Read the model definition and answer for the solid it produces. Units are mm, in the model's axes. A direction names the side the tool comes from. Give positions to 0.01 mm unless a question says otherwise; leave off trailing zeros. Order: outer loops, then holes, each group sorted by start corner. A loop starts at its lowest first (then second) coordinate and runs counter-clockwise, first axis right, second up. Notation, with made-up numbers: M 64,22.25 L 71,22.25 A32 ccw 71,51.25 Z; hole C -23.75,-14 d11. An arc over 180 degrees is marked long. One line per item, written item: value.
from build123d import *

# Parameters (mm, degrees)
SKETCH1_W                = 4
SKETCH1_H                = 15
BOSS_EXTRUDE1_DEPTH      = 4
SKETCH2_R                = 0.925
BOSS_EXTRUDE2_DEPTH      = 2
BOSS_EXTRUDE2_DEPTH_BACK = 17
CHAMFER1_SIZE            = 0.5
BOSS_EXTRUDE3_DEPTH      = 2
BOSS_EXTRUDE4_DEPTH      = 2


with BuildPart() as part:
    # Sketch1 → Boss-Extrude1 (new body)
    with BuildSketch(Plane(origin=(0, 0, 0), x_dir=(1, 0, 0), z_dir=(0, 1, 0))):
        Rectangle(SKETCH1_W, SKETCH1_H)
    extrude(amount=BOSS_EXTRUDE1_DEPTH)

    # Sketch2 → Boss-Extrude2 (add, two sides)
    with BuildSketch(Plane.XY.offset(7.5)) as boss_extrude2_sk:
        with Locations((0, 2)):
            Circle(SKETCH2_R)
    extrude(amount=BOSS_EXTRUDE2_DEPTH)
    extrude(boss_extrude2_sk.sketch, amount=-BOSS_EXTRUDE2_DEPTH_BACK)

    # Chamfer1
    chamfer1_edges = [part.edges().sort_by_distance(p)[0] for p in [
        (-2, 4, 0),
        (2, 4, 0),
        (-2, 0, 0),
        (2, 0, 0),
    ]]
    chamfer(chamfer1_edges, length=CHAMFER1_SIZE)

    # Sketch3 → Boss-Extrude3 (add)
    with BuildSketch(Plane.XY.offset(9.5)):
        with BuildLine():
            Line((-0.75, 2.925), (0.75, 2.925))
            ThreePointArc((0.75, 2.925), (1.675, 2), (0.75, 1.075))
            Line((0.75, 1.075), (-0.75, 1.075))
            ThreePointArc((-0.75, 1.075), (-1.675, 2), (-0.75, 2.925))
        make_face()
    extrude(amount=BOSS_EXTRUDE3_DEPTH)

    # Sketch4 → Boss-Extrude4 (add)
    with BuildSketch(Plane(origin=(0, 0, -9.5), x_dir=(-1, 0, 0), z_dir=(0, 0, -1))):
        with BuildLine():
            Line((-0.75, 2.925), (0.75, 2.925))
            ThreePointArc((0.75, 2.925), (1.675, 2), (0.75, 1.075))
            Line((0.75, 1.075), (-0.75, 1.075))
            ThreePointArc((-0.75, 1.075), (-1.675, 2), (-0.75, 2.925))
        make_face()
    extrude(amount=BOSS_EXTRUDE4_DEPTH)


solid = part.part
1) Consider probe 1 along Z at (x, y) = (-1.55, 2); probe 2 along Z at (x, y) = (-1.1, 0.75); probe 3 along X at (y, z) = (1.95, -8.5). Determine where each line is inside the solid, lowest interval first.
Reported:
probe 1: z = -11.5 to -9.5, -7.5 to 7.5, 9.5 to 11.5
probe 2: z = -7.5 to 7.5
probe 3: x = -0.92 to 0.92
2) Determine the mould class of faces 1 (the face through (-1.2, 2, 9.5)), 2 (the face through (0, 2, 11.5)), 3 (the face through (-0.12, 2.917, -8.486)), 4 (the face through (0, 1.075, -10)) for opening direction Z: +Z half, -Z half, draft (parallel to the pull), parting line (faces both ways), or undercut.
Reported:
face 1: undercut
face 2: +Z half
face 3: undercut
face 4: draft
3) Find section C-C, the plane x = 0.4. Write down the section's boundary in (y, z) (3 decimals).
Reported:
outline: M 0,-7.5 L 1.166,-7.5 L 1.166,-9.5 L 1.075,-9.5 L 1.075,-11.5 L 2.925,-11.5 L 2.925,-9.5 L 2.834,-9.5 L 2.834,-7.5 L 4,-7.5 L 4,7.5 L 2.834,7.5 L 2.834,9.5 L 2.925,9.5 L 2.925,11.5 L 1.075,11.5 L 1.075,9.5 L 1.166,9.5 L 1.166,7.5 L 0,7.5 Z
4) Find section D-D, the plane z = -10. Write down the section's boundary in (x, y) (3 decimals).
Reported:
outline: M -0.75,1.075 L 0.75,1.075 A0.925 ccw 0.75,2.925 L -0.75,2.925 A0.925 ccw Z
5) Each of these flat-tipped pins is pushed along its axis until it touches: pin 1 Ø1.2 at (x, z) = (0, 11) entering from -Y (3 decimals); pin 2 Ø1.6 at (x, z) = (0.5, 10) entering from +Y (3 decimals). Where does it stop, or does it pass through?
Reported:
pin 1: stops at y = 1.075
pin 2: stops at y = 2.925
6) Find section A-A, the plane y = 2. Write down the section's boundary in (x, z) (3 decimals), plus the area to 3 significant figures.
Reported:
outline: M -2,-7.5 L -0.925,-7.5 L -0.925,-9.5 L -1.675,-9.5 L -1.675,-11.5 L 1.675,-11.5 L 1.675,-9.5 L 0.925,-9.5 L 0.925,-7.5 L 2,-7.5 L 2,7.5 L 0.925,7.5 L 0.925,9.5 L 1.675,9.5 L 1.675,11.5 L -1.675,11.5 L -1.675,9.5 L -0.925,9.5 L -0.925,7.5 L -2,7.5 Z
area: 80.8 mm^2
7) Find section B-B, the plane z = 0.25. Write down the section's boundary in (x, y), plus the area to 3 significant figures.
Reported:
outline: M -2,0.5 L -1.5,0 L 1.5,0 L 2,0.5 L 2,3.5 L 1.5,4 L -1.5,4 L -2,3.5 Z
area: 15.5 mm^2
8) Which of the six approach directions +Z, -Z, +X, -X, +Y, -Y give full straight-line access (tool end or side, diameter ignored) to faces 5 (the face through (0, 2.925, -10)), 6 (the face through (-1.675, 2.02, -10.486)), 7 (the face through (1.675, 2.02, 10.486))?
Reported:
face 5: -Z, +X, -X, +Y
face 6: -Z, -X
face 7: +Z, +X
